```python
from build123d import *

# Parameters (mm, degrees)
SKETCH_5_R               = 9
CUT_EXTRUDE_1_DEPTH      = 59.060313468
PATTERN_CIRCULAR_1_COUNT = 9


with BuildPart() as part:
    # 草图4 → 旋转1 (revolve)
    with BuildSketch(Plane(origin=(0, 0, 0), x_dir=(0, 0, -1), z_dir=(1, 0, 0))):
        with BuildLine():
            Line((0, 17.370620624), (0, 41))
            Line((0, 41), (3, 41))
            Line((3, 41), (3, 19.849287907))
            ThreePointArc((3, 19.849287907), (4.519902914, 19.393505195), (6, 18.821530225))
            Line((6, 18.821530225), (6, 15.5))
            ThreePointArc((6, 15.5), (3.084663444, 16.706867601), (0, 17.370620624))
        make_face()
    revolve(axis=Axis((0, 0, 0), (0, 0, -1)))

    # 草图5 → 切除-拉伸1 (cut, through all)
    with BuildSketch(Plane(origin=(0, 0, -3), x_dir=(-1, 0, 0), z_dir=(0, 0, -1))):
        with Locations((0, 29.5)):
            Circle(SKETCH_5_R)
    cut_extrude_1 = extrude(amount=-CUT_EXTRUDE_1_DEPTH, mode=Mode.SUBTRACT)

    # 阵列(圆周)1: 切除-拉伸1 ×9 about axis
    pattern_circular_1_axis = Axis((0, 0, 0), (0, 0, 1))
    for i in range(1, PATTERN_CIRCULAR_1_COUNT):
        add(cut_extrude_1.rotate(pattern_circular_1_axis, i * 360 / PATTERN_CIRCULAR_1_COUNT), mode=Mode.SUBTRACT)


solid = part.part
```
Part model, mm, in its own coordinate system. A direction names the side the tool comes from. Give positions to 0.01 mm unless a question says otherwise; leave off trailing zeros. Order: outer loops, then holes, each group sorted by start corner. A loop starts at its lowest first (then second) coordinate and runs counter-clockwise, first axis right, second up. Notation, with made-up numbers: M 15.5,58 L 49.5,58 A19 cw 49.5,92 Z; hole C 16.5,22 d11. An arc over 180 degrees is marked long. Use a Markdown table: item, result. Add a question column.
(1) Saw through at C-C, the plane y = -35. Give the cut face in (x, z), and give its area (3 significant figures).
(2) Probe line 1 along X through (y, z) = (-20.5, -1); line 2 along Y through (x, z) = (0.5, -1); line 3 along X through (y, z) = (-27.5, -1.25). List the from-to ranges inside material, lowest first. Write a range as [from, to].
(3) Mould opens along Y. For faces 3 (the face through (-40, -9, -2)), 4 (the face through (20.738, 1.676, -1.521)), 5 (the face through (-12.33, 28.68, -1.52)), 6 (the face through (14, -7.1, -6)) say: +Y half, -Y half, draft (parallel to the pull), parting line (faces both ways), or undercut.
(4) Saw through at B-B, the plane y = 9. Give the cut face in (x, z), and give its area (3 significant figures).
(5) 3-axis set-ups, long thin cutter, end or side, ignore diameter. For faces 1 (the face through (17.234, -18.197, -1.521)), 2 (the face through (-18, -9, -3)): which of +Z, -Z, +X, -X, +Y, -Y reach the whole face in a straight line?
(6) Drop flat-ended pins along their axis: P1, Ø1, axis at y = 6.5, z = -2.5, coming from the -X side; P2, Ø1.5, axis at x = 12.5, z = -4.5, coming from the +Y side; P3, Ø2, axis at y = 12, z = -2.5, coming from the -X side. Give the stop position or say it passes through.
(7) Saw through at D-D, the plane x = -23.5. Give the cut face in (y, z), and give its area (3 significant figures).
(8) Saw through at A-A, the plane x = 0. Give the cut face in (y, z), and give its area (3 significant figures).
Answer key:
| question | item | result |
|---|---|---|
| 1 | outline | M -21.35,-3 L -15.38,-3 L -15.38,0 L -21.35,0 Z; M -4.8,-3 L 4.8,-3 L 4.8,0 L -4.8,0 Z; M 15.38,-3 L 21.35,-3 L 21.35,0 L 15.38,0 Z |
| 1 | area | 64.6 mm^2 |
| 2 | line 1 | [-35.51, -32.47], [-18.62, -15.46], [-4.72, 4.72], [15.46, 18.62], [32.47, 35.51] |
| 2 | line 2 | [-41, -17.21], [17.21, 20.51], [38.49, 41] |
| 2 | line 3 | [-30.41, -19.09], [-1.09, 1.09], [19.09, 30.41] |
| 3 | face 3 | parting line |
| 3 | face 4 | undercut |
| 3 | face 5 | undercut |
| 3 | face 6 | draft |
| 4 | outline | M -40,-3 L -37.17,-3 L -37.17,0 L -40,0 Z; M -20.93,-3 L -17.69,-3 A18.42 ccw -16.53,-6 L -12.62,-6 A15.01 cw -14.86,0 L -20.93,0 Z; M 12.62,-6 L 16.53,-6 A18.42 ccw 17.69,-3 L 20.93,-3 L 20.93,0 L 14.86,0 A15.01 cw Z; M 37.17,-3 L 40,-3 L 40,0 L 37.17,0 Z |
| 4 | area | 77.7 mm^2 |
| 5 | face 1 | +Z, -Z |
| 5 | face 2 | -Z |
| 6 | P1 | x = -40.56 |
| 6 | P2 | y = 15.52 |
| 6 | P3 | x = -39.5 |
| 7 | outline | M -33.6,-3 L -23.51,-3 L -23.51,0 L -33.6,0 Z; M -5.99,-3 L -1.96,-3 L -1.96,0 L -5.99,0 Z; M 12.21,-3 L 14.83,-3 L 14.83,0 L 12.21,0 Z; M 30.37,-3 L 33.6,-3 L 33.6,0 L 30.37,0 Z |
| 7 | area | 59.9 mm^2 |
| 8 | outline | M -41,-3 L -19.85,-3 A20.5 ccw -18.82,-6 L -15.5,-6 A17.5 cw -17.37,0 L -41,0 Z; M 15.5,-6 L 18.82,-6 A20.5 ccw 19.85,-3 L 20.5,-3 L 20.5,0 L 17.37,0 A17.5 cw Z; M 38.5,-3 L 41,-3 L 41,0 L 38.5,0 Z |
| 8 | area | 109 mm^2 |
